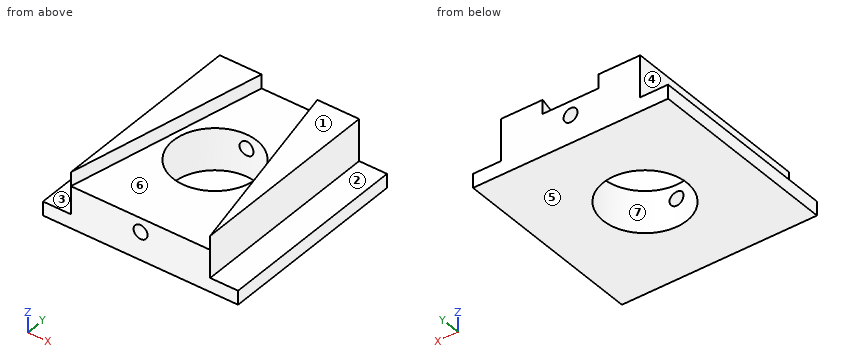
```python
from build123d import *

# Parameters (mm, degrees)
F0_W     = 177.8
F0_H     = 177.8
F0_R     = 38.1
F1_DEPTH = 38.1
F2_W     = 25.4
F2_H     = 177.8
F3_DEPTH = 25.4
F4_R     = 6.35
F5_DEPTH = 177.801
F7_DEPTH = 12.7


with BuildPart() as f1:
    # F0 (on Top) → F1 (new body)
    with BuildSketch(Plane.XY):
        Rectangle(F0_W, F0_H)
        Circle(F0_R, mode=Mode.SUBTRACT)
    extrude(amount=F1_DEPTH)

    # F2 (on face) → F3 (cut)
    with BuildSketch(Plane.XY.offset(38.1)):
        with Locations((-76.2, 0)):
            Rectangle(F2_W, F2_H)
        with Locations((76.2, 0)):
            Rectangle(F2_W, F2_H)
    extrude(amount=-F3_DEPTH, mode=Mode.SUBTRACT)

    # F4 (on face) → F5 (cut, through all)
    with BuildSketch(Plane.XZ.offset(88.9)):
        with Locations((0, 25.4)):
            Circle(F4_R)
    extrude(amount=-F5_DEPTH, mode=Mode.SUBTRACT)

    # F6 (on face) → F7 (join)
    with BuildSketch(Plane.XY.offset(38.1)):
        Polygon((63.5, 88.9), (25.4, 88.9), (63.5, -88.9), align=None)
        Polygon((-63.5, -88.9), (-25.4, 88.9), (-63.5, 88.9), align=None)
    extrude(amount=F7_DEPTH)


solid = f1.part
```
Geometry check sheet. Reference: the model listing, model coordinates, mm. Face numbers are marked on the shaded views. A direction names the side the tool comes from. Give positions to 0.01 mm unless a question says otherwise; leave off trailing zeros. Order: outer loops, then holes, each group sorted by start corner. A loop starts at its lowest first (then second) coordinate and runs counter-clockwise, first axis right, second up.
1. Gauge pin test, flat ends, axial feed: pin 1 Ø10 at (x, z) = (0, 25.4) entering from +Y; pin 2 Ø19 at (y, z) = (42, 30) entering from +X; pin 3 Ø1 at (x, y) = (-3, -68.5) entering from +Z; pin 4 Ø1.5 at (y, z) = (-15.5, 22) entering from -X. Record the tip position at first contact, or that the pin passes through.
2. Thickness scan on L1, parallel to X at y = -62.5, z = 25.5; L2, parallel to Z at x = 0, y = 67; L3, parallel to Z at x = 48, y = -23. Record the ranges inside material, lowest first.
3. Section check A-A, the plane z = 25.4. Enter the section's corners in (x, y).
4. Section check D-D, the plane y = -65.5. Enter the section's corners in (x, z).
5. Release check for a two-part mould opening along X. For the marked faces 4, 5, 6 and 7 record: pulls with the +X half, pulls with the -X half, needs draft (parallel to the pull), parting line crosses it, or undercut.
6. Access from +Z, -Z, +X, -X, +Y, -Y to the whole of each face (thin tool, end or side, straight path). Record for the marked faces 1, 2 and 3.
7. Section check C-C, the plane x = -18. Enter the section's corners in (y, z).
8. Section check B-B, the plane x = 0. Enter the section's corners in (y, z), and give its area (3 significant figures).
Values follow:
1. pin 1: passes through
1. pin 2: stops at x = 63.5
1. pin 3: stops at z = 38.1
1. pin 4: stops at x = -63.5
2. L1: x = -63.5 to -6.35, 6.35 to 63.5
2. L2: z = 0 to 19.05, 31.75 to 38.1
2. L3: z = 0 to 38.1
3. outline: (-63.5, -88.9) - (-6.35, -88.9) - (-6.35, -37.57) arc R38.1 cw to (-6.35, 37.57) - (-6.35, 88.9) - (-63.5, 88.9) - close; (6.35, -88.9) - (63.5, -88.9) - (63.5, 88.9) - (6.35, 88.9) - (6.35, 37.57) arc R38.1 cw to (6.35, -37.57) - close
4. outline: (-88.9, 0) - (88.9, 0) - (88.9, 12.7) - (63.5, 12.7) - (63.5, 50.8) - (58.49, 50.8) - (58.49, 38.1) - (-58.49, 38.1) - (-58.49, 50.8) - (-63.5, 50.8) - (-63.5, 12.7) - (-88.9, 12.7) - close; hole circle Ø12.7 at (0, 25.4)
5. face 4: pulls with the -X half
5. face 5: needs draft
5. face 6: undercut
5. face 7: undercut
6. face 1: +Z, +X, -X, +Y, -Y
6. face 2: +Z, +X, +Y, -Y
6. face 3: +Z, -X, +Y, -Y
7. outline: (-88.9, 0) - (-33.58, 0) - (-33.58, 38.1) - (-88.9, 38.1) - close; (33.58, 0) - (88.9, 0) - (88.9, 38.1) - (33.58, 38.1) - close
8. outline: (-88.9, 0) - (-38.1, 0) - (-38.1, 19.05) - (-88.9, 19.05) - close; (-88.9, 31.75) - (-38.1, 31.75) - (-38.1, 38.1) - (-88.9, 38.1) - close; (38.1, 0) - (88.9, 0) - (88.9, 19.05) - (38.1, 19.05) - close; (38.1, 31.75) - (88.9, 31.75) - (88.9, 38.1) - (38.1, 38.1) - close
8. area: 2,580 mm2
